Could you check a few things on this model? Use its own coordinates, in mm. A direction names the side the tool comes from. Give positions to 0.01 mm unless a question says otherwise; leave off trailing zeros. Order: outer loops, then holes, each group sorted by start corner. A loop starts at its lowest first (then second) coordinate and runs counter-clockwise, first axis right, second up. Notation, with made-up numbers: M 67,64.25 L 99,64.25 A34 cw 99,102.25 Z; hole C 75.5,49.25 d5. An arc over 180 degrees is marked long. Use a Markdown table: item, result. Add a question column.
Item 1: Suppose I cut it at A-A on z = 0. Write out the boundary of the cut face in (x, y).
Item 2: If we mould it in two halves opening along X, with no side actions, what happens to faces 1 (the face through (83.4, 0, -0.4)), 2 (the face through (-47.5, 3, 5.4)), 3 (the face through (-91.5, 1, 0.1))? For each: released by +X, released by -X, zero draft, split by the parting line, or undercut.
Item 3: If I drill on L1, parallel to Z at x = -85, y = -0.15; L2, parallel to X at y = 0, z = 0; L3, parallel to X at y = 1.5, z = -0.25, over which ranges is the centre line in solid material (lowest first)? Write a range as from..to.
Item 4: Suppose I cut it at B-B on x = 78. Write out the boundary of the cut face in (y, z).
Item 5: For faces 4 (the face through (51.1, 3, -5.5)), 5 (the face through (-3.9, 5, 6)), 6 (the face through (-1, 1, -6.5)), 7 (the face through (50, 1, 6.5)), 8 (the face through (-49, 1, 6.5)), which set-ups out of +Z, -Z, +X, -X, +Y, -Y let a thin tool reach every point of the face, with its end or its side?
Item 6: I'm going to push flat-ended pins straight in: pin 1 Ø1.5 at (x, z) = (-48.5, -1.5) entering from +Y; pin 2 Ø10 at (x, z) = (-67.5, -0.5) entering from +Y; pin 3 Ø2.5 at (y, z) = (6, 8) entering from +X; pin 4 Ø3 at (x, y) = (-51.5, 1) entering from +Z. Where does each tip first touch, or does it pass through?
from build123d import *

# Parameters (mm, degrees)
SKETCH1_R               = 1.65
BOSS_EXTRUDE1_DEPTH     = 1
SKETCH2_W               = 7.8
SKETCH2_H               = 13
BOSS_EXTRUDE2_DEPTH     = 10
BOSS_EXTRUDE3_DEPTH     = 7.8
CUT_EXTRUDE1_DEPTH      = 97.907997606
CUT_EXTRUDE1_DEPTH_BACK = 97.907997606
SKETCH4_R               = 1.65
SKETCH7_W               = 8
SKETCH7_H               = 6.5
BOSS_EXTRUDE5_DEPTH     = 2
FILLET3_R               = 2
BOSS_EXTRUDE4_DEPTH     = 2
CUT_EXTRUDE2_DEPTH      = 10
FILLET1_R               = 5
FILLET2_R               = 2


with BuildPart() as part:
    # Sketch1 → Boss-Extrude1 (new, symmetric)
    with BuildSketch(Plane(origin=(0, 0, 0), x_dir=(1, 0, 0), z_dir=(0, 1, 0))):
        with BuildLine():
            Line((-85, 6.5), (85, 6.5))
            ThreePointArc((85, 6.5), (91.5, 0), (85, -6.5))
            Line((85, -6.5), (-85, -6.5))
            ThreePointArc((-85, -6.5), (-91.5, 0), (-85, 6.5))
        make_face()
        with Locations(Location((-85, 0, 0), (0, 0, 270))):
            Circle(SKETCH1_R, mode=Mode.SUBTRACT)
        with Locations(Location((85, 0, 0), (0, 0, 270))):
            Circle(SKETCH1_R, mode=Mode.SUBTRACT)
    extrude(amount=BOSS_EXTRUDE1_DEPTH, both=True)

    # Sketch2 → Boss-Extrude2 (add)
    with BuildSketch(Plane(origin=(0, 1, 0), x_dir=(1, 0, 0), z_dir=(0, 1, 0))):
        Rectangle(SKETCH2_W, SKETCH2_H)
    extrude(amount=BOSS_EXTRUDE2_DEPTH)

    # Sketch3 → Boss-Extrude3 (add)
    with BuildSketch(Plane(origin=(3.9, 0, 0), x_dir=(0, 0, -1), z_dir=(1, 0, 0))):
        with BuildLine():
            Line((-6.5, 11), (-8, 11))
            ThreePointArc((-8, 11), (-11.535533906, 9.535533906), (-13, 6))
            Line((-13, 6), (-13, -1))
            Line((-13, -1), (-6.5, -1))
            Line((-6.5, -1), (-6.5, 11))
        make_face()
    extrude(amount=-BOSS_EXTRUDE3_DEPTH)

    # Sketch4 → Cut-Extrude1 (cut, two sides: drawn at the far end of the back side and taken through both)
    with BuildSketch(Plane(origin=(3.9, 0, 0), x_dir=(0, 0, -1), z_dir=(1, 0, 0)).offset(-CUT_EXTRUDE1_DEPTH_BACK)):
        with Locations((-8, 6)):
            Circle(SKETCH4_R)
    extrude(amount=CUT_EXTRUDE1_DEPTH + CUT_EXTRUDE1_DEPTH_BACK, mode=Mode.SUBTRACT)

    # Sketch7 → Boss-Extrude5 (add)
    with BuildSketch(Plane(origin=(0, 1, 0), x_dir=(1, 0, 0), z_dir=(0, 1, 0))):
        with Locations((-7.9, -9.75)):
            Rectangle(SKETCH7_W, SKETCH7_H)
        with Locations((7.9, -9.75)):
            Rectangle(SKETCH7_W, SKETCH7_H)
    extrude(amount=-BOSS_EXTRUDE5_DEPTH)

    # Fillet3
    fillet3_edges = [part.edges().sort_by_distance(p)[0] for p in [
        (-11.9, 0, 6.5),
        (-11.9, 0, 13),
        (11.9, 0, 6.5),
        (11.9, 0, 13),
    ]]
    fillet(fillet3_edges, radius=FILLET3_R)

    # Sketch5 → Boss-Extrude4 (add)
    with BuildSketch(Plane(origin=(0, 1, 0), x_dir=(1, 0, 0), z_dir=(0, 1, 0))):
        with BuildLine():
            Line((-85, 6.5), (85, 6.5))
            ThreePointArc((85, 6.5), (91.5, 0), (85, -6.5))
            Line((85, -6.5), (13.9, -6.5))
            ThreePointArc((13.9, -6.5), (12.485786438, -7.085786438), (11.9, -8.5))
            Line((11.9, -8.5), (11.9, -11))
            ThreePointArc((11.9, -11), (11.314213562, -12.414213562), (9.9, -13))
            Line((9.9, -13), (-9.9, -13))
            ThreePointArc((-9.9, -13), (-11.314213562, -12.414213562), (-11.9, -11))
            Line((-11.9, -11), (-11.9, -8.5))
            ThreePointArc((-11.9, -8.5), (-12.485786438, -7.085786438), (-13.9, -6.5))
            Line((-13.9, -6.5), (-85, -6.5))
            ThreePointArc((-85, -6.5), (-91.5, 0), (-85, 6.5))
        make_face()
        with BuildLine():
            Line((-85, 5), (85, 5))
            ThreePointArc((85, 5), (90, 0), (85, -5))
            Line((85, -5), (13.9, -5))
            ThreePointArc((13.9, -5), (11.425126266, -6.025126266), (10.4, -8.5))
            Line((10.4, -8.5), (10.4, -11))
            ThreePointArc((10.4, -11), (10.253553391, -11.353553391), (9.9, -11.5))
            Line((9.9, -11.5), (-9.9, -11.5))
            ThreePointArc((-9.9, -11.5), (-10.253553391, -11.353553391), (-10.4, -11))
            Line((-10.4, -11), (-10.4, -8.5))
            ThreePointArc((-10.4, -8.5), (-11.425126266, -6.025126266), (-13.9, -5))
            Line((-13.9, -5), (-85, -5))
            ThreePointArc((-85, -5), (-90, 0), (-85, 5))
        make_face(mode=Mode.SUBTRACT)
    extrude(amount=BOSS_EXTRUDE4_DEPTH)

    # Sketch6 → Cut-Extrude2 (cut)
    with BuildSketch(Plane.ZY.offset(3.9)):
        Polygon((-6.5, 3), (6.5, 11), (-6.5, 11), align=None)
    extrude(amount=-CUT_EXTRUDE2_DEPTH, mode=Mode.SUBTRACT)

    # Fillet1
    fillet1_edges = [part.edges().sort_by_distance(p)[0] for p in [
        (0, 11, 6.5),
    ]]
    fillet(fillet1_edges, radius=FILLET1_R)

    # Fillet2
    fillet2_edges = [part.edges().sort_by_distance(p)[0] for p in [
        (-3.9, 2, -5),
        (3.9, 2, -5),
    ]]
    fillet(fillet2_edges, radius=FILLET2_R)


solid = part.part
Findings below:
| question | item | result |
|---|---|---|
| 1 | outline | M -91.5,-1 L -86.65,-1 L -86.65,1 L -90,1 L -90,3 L -91.5,3 Z; M -83.35,-1 L 83.35,-1 L 83.35,1 L 3.9,1 L 3.9,7 L -3.9,7 L -3.9,1 L -83.35,1 Z; M 86.65,-1 L 91.5,-1 L 91.5,3 L 90,3 L 90,1 L 86.65,1 Z |
| 2 | face 1 | undercut |
| 2 | face 2 | zero draft |
| 2 | face 3 | released by -X |
| 3 | L1 | z = -6.5..-1.65, 1.65..6.5 |
| 3 | L2 | x = -91.5..-86.65, -83.35..83.35, 86.65..91.5 |
| 3 | L3 | x = -91.5..-89.99, -3.9..3.9, 89.99..91.5 |
| 4 | outline | M -1,-6.5 L 3,-6.5 L 3,-5 L 1,-5 L 1,5 L 3,5 L 3,6.5 L -1,6.5 Z |
| 5 | face 4 | +Z, -Z, +X, +Y |
| 5 | face 5 | +Y |
| 5 | face 6 | -Z, +X, -X, +Y, -Y |
| 5 | face 7 | +Z, +X, +Y, -Y |
| 5 | face 8 | +Z, -X, +Y, -Y |
| 6 | pin 1 | stops at y = 1 |
| 6 | pin 2 | stops at y = 3 |
| 6 | pin 3 | passes through |
| 6 | pin 4 | stops at z = 6.5 |
